from build123d import *

# Parameters (mm, degrees)
SKETCH1_W           = 100
SKETCH1_H           = 60
BOSS_EXTRUDE1_DEPTH = 3
SKETCH2_R           = 2
SKETCH2_R_2         = 1.5
CUT_EXTRUDE1_DEPTH  = 59.386642308
FILLET1_R           = 1


with BuildPart() as part:
    # Sketch1 → Boss-Extrude1 (new body)
    with BuildSketch(Plane(origin=(0, 0, 0), x_dir=(1, 0, 0), z_dir=(0, 1, 0))):
        Rectangle(SKETCH1_W, SKETCH1_H)
    extrude(amount=BOSS_EXTRUDE1_DEPTH)

    # Sketch2 → Cut-Extrude1 (cut, through all)
    with BuildSketch(Plane(origin=(0, 3, 0), x_dir=(1, 0, 0), z_dir=(0, 1, 0))):
        with BuildLine():
            Line((-45, 1.5), (-24.242640687, 1.5))
            ThreePointArc((-24.242640687, 1.5), (-23.181980515, 3.181980515), (-21.5, 4.242640687))
            Line((-21.5, 4.242640687), (-21.5, 25))
            Line((-21.5, 25), (-45, 25))
            Line((-45, 25), (-45, 1.5))
        make_face()
        with BuildLine():
            Line((-45, -1.5), (-45, -25))
            Line((-45, -25), (-21.5, -25))
            Line((-21.5, -25), (-21.5, -4.242640687))
            ThreePointArc((-21.5, -4.242640687), (-23.181980515, -3.181980515), (-24.242640687, -1.5))
            Line((-24.242640687, -1.5), (-45, -1.5))
        make_face()
        with BuildLine():
            Line((-18.5, 25), (-18.5, 4.242640687))
            ThreePointArc((-18.5, 4.242640687), (-16.818019485, 3.181980515), (-15.757359313, 1.5))
            Line((-15.757359313, 1.5), (5.757359313, 1.5))
            ThreePointArc((5.757359313, 1.5), (6.818019485, 3.181980515), (8.5, 4.242640687))
            Line((8.5, 4.242640687), (8.5, 25))
            Line((8.5, 25), (-18.5, 25))
        make_face()
        with BuildLine():
            ThreePointArc((-15.757359313, -1.5), (-16.818019485, -3.181980515), (-18.5, -4.242640687))
            Line((-18.5, -4.242640687), (-18.5, -25))
            Line((-18.5, -25), (8.5, -25))
            Line((8.5, -25), (8.5, -4.242640687))
            ThreePointArc((8.5, -4.242640687), (6.818019485, -3.181980515), (5.757359313, -1.5))
            Line((5.757359313, -1.5), (-15.757359313, -1.5))
        make_face()
        with BuildLine():
            ThreePointArc((14.242640687, -1.5), (13.181980515, -3.181980515), (11.5, -4.242640687))
            Line((11.5, -4.242640687), (11.5, -25))
            Line((11.5, -25), (28.5, -25))
            Line((28.5, -25), (28.5, -4.242640687))
            ThreePointArc((28.5, -4.242640687), (26.818019485, -3.181980515), (25.757359313, -1.5))
            Line((25.757359313, -1.5), (14.242640687, -1.5))
        make_face()
        with BuildLine():
            Line((11.5, 25), (11.5, 4.242640687))
            ThreePointArc((11.5, 4.242640687), (13.181980515, 3.181980515), (14.242640687, 1.5))
            Line((14.242640687, 1.5), (25.757359313, 1.5))
            ThreePointArc((25.757359313, 1.5), (26.818019485, 3.181980515), (28.5, 4.242640687))
            Line((28.5, 4.242640687), (28.5, 25))
            Line((28.5, 25), (11.5, 25))
        make_face()
        with BuildLine():
            Line((31.5, 25), (31.5, 4.242640687))
            ThreePointArc((31.5, 4.242640687), (33.181980515, 3.181980515), (34.242640687, 1.5))
            Line((34.242640687, 1.5), (45, 1.5))
            Line((45, 1.5), (45, 25))
            Line((45, 25), (31.5, 25))
        make_face()
        with BuildLine():
            ThreePointArc((34.242640687, -1.5), (33.181980515, -3.181980515), (31.5, -4.242640687))
            Line((31.5, -4.242640687), (31.5, -25))
            Line((31.5, -25), (45, -25))
            Line((45, -25), (45, -1.5))
            Line((45, -1.5), (34.242640687, -1.5))
        make_face()
        with Locations(Location((30, 0, 0), (0, 0, 270))):
            Circle(SKETCH2_R)
        with Locations(Location((10, 0, 0), (0, 0, 270))):
            Circle(SKETCH2_R)
        with Locations(Location((-20, 0, 0), (0, 0, 270))):
            Circle(SKETCH2_R)
        with Locations(Location((-47, -27, 0), (0, 0, 270))):
            Circle(SKETCH2_R_2)
        with Locations(Location((-47, 27, 0), (0, 0, 270))):
            Circle(SKETCH2_R_2)
        with Locations(Location((47, -27, 0), (0, 0, 270))):
            Circle(SKETCH2_R_2)
        with Locations(Location((47, 27, 0), (0, 0, 270))):
            Circle(SKETCH2_R_2)
    extrude(amount=-CUT_EXTRUDE1_DEPTH, mode=Mode.SUBTRACT)

    # Fillet1
    fillet1_edges = [part.edges().sort_by_distance(p)[0] for p in [
        (8.5, 1.5, 25),
        (-18.5, 1.5, 25),
        (28.5, 1.5, 25),
        (11.5, 1.5, 25),
        (-45, 1.5, -1.5),
        (-45, 1.5, -25),
        (-21.5, 1.5, -25),
        (11.5, 1.5, -25),
        (31.5, 1.5, -25),
        (45, 1.5, -25),
        (45, 1.5, -1.5),
        (45, 1.5, 1.5),
        (45, 1.5, 25),
        (31.5, 1.5, 25),
        (-21.5, 1.5, 25),
        (-45, 1.5, 25),
        (-45, 1.5, 1.5),
        (-18.5, 1.5, -25),
        (8.5, 1.5, -25),
    ]]
    fillet(fillet1_edges, radius=FILLET1_R)


solid = part.part
Part model, mm, in its own coordinate system. Coordinates: 2 decimals unless noted, no trailing zeros. Write each loop counter-clockwise with the first axis right and the second up, starting at its lowest first coordinate (ties: lowest second). Pieces come first, ordered by that corner, then holes. Notation, with made-up numbers: (74, -22.75) - (114, -22.75) arc R14 cw to (114, -3.75) - close; hole circle Ø8 at (4.5, 28.25). An arc over 180 degrees is marked (long way). Put each result on its own line as item: value.
1. Probe line 1 along Z through (x, y) = (-34.5, 2.45); line 2 along X through (y, z) = (0.55, 22); line 3 along X through (y, z) = (0.7, 0). List the from-to ranges inside material, lowest first. Write a range as [from, to].
Final values:
line 1: z = [-30, -25], [-1.5, 1.5], [25, 30]
line 2: x = [-50, -45], [-21.5, -18.5], [8.5, 11.5], [28.5, 31.5], [45, 50]
line 3: x = [-50, -22], [-18, 8], [12, 28], [32, 50]
2. Band-saw the part on B-B (z = -27). Write the cut outline in (x, y).
Final values:
outline: (-50, 0) - (-48.5, 0) - (-48.5, 3) - (-50, 3) - close; (-45.5, 0) - (45.5, 0) - (45.5, 3) - (-45.5, 3) - close; (48.5, 0) - (50, 0) - (50, 3) - (48.5, 3) - close
3. Band-saw the part on D-D (x = 30). Write the cut outline in (y, z).
Final values:
outline: (0, -30) - (3, -30) - (3, -2) - (0, -2) - close; (0, 2) - (3, 2) - (3, 30) - (0, 30) - close
4. Band-saw the part on A-A (x = -47). Write the cut outline in (y, z), then the cut area to 3 significant figures.
Final values:
outline: (0, -30) - (3, -30) - (3, -28.5) - (0, -28.5) - close; (0, -25.5) - (3, -25.5) - (3, 25.5) - (0, 25.5) - close; (0, 28.5) - (3, 28.5) - (3, 30) - (0, 30) - close
area: 162 mm²
5. Two-plate mould, pull along Z, no slides. Class faces 1 (the cylindrical face through (45.536, 1.521, -27.325)), 2 (the flat face through (-1, 3, 0)): +Z half, -Z half, draft (parallel to the pull), parting line (faces both ways), or undercut.
Final values:
face 1: undercut
face 2: draft
6. Band-saw the part on C-C (z = 0). Write the cut outline in (x, y), then the cut area to 3 significant figures.
Final values:
outline: (-50, 0) - (-22, 0) - (-22, 3) - (-50, 3) - close; (-18, 0) - (8, 0) - (8, 3) - (-18, 3) - close; (12, 0) - (28, 0) - (28, 3) - (12, 3) - close; (32, 0) - (50, 0) - (50, 3) - (32, 3) - close
area: 264 mm²
